For this review, take the finished solid that the model builds, in its own axes (mm). Face numbers are marked on the shaded views. A direction names the side the tool comes from. Give positions to 0.01 mm unless a question says otherwise; leave off trailing zeros. Order: outer loops, then holes, each group sorted by start corner. A loop starts at its lowest first (then second) coordinate and runs counter-clockwise, first axis right, second up. Notation, with made-up numbers: M 41.25,74.25 L 62.25,74.25 A6 ccw 62.25,79.25 Z; hole C 25,53 d3. An arc over 180 degrees is marked long. Answer as CSV lines item,"result". Start each with the question number.
1. For line 1 along Z through (x, y) = (18, -24); line 2 along Y through (x, z) = (18, 5); line 3 along Z through (x, y) = (-8.5, 7), list the stretches that pass through material, from the lowest coordinate up.
2. We need section D-D, the plane y = 27.5. Give the boundary of the cut face in (x, z).
3. Machinability: for the marked faces 5, 6 and 7, which of the approach directions +Z, -Z, +X, -X, +Y, -Y give a long, thin tool a straight path to every point of the face, cutting with its end or side? Answer none if there is none.
4. We need section C-C, the plane z = 5. Give the boundary of the cut face in (x, y), and give its area (3 significant figures).
5. Mouldability with a two-part tool opening along Z and no side actions: class the marked faces 1, 2, 3 and 4 as pulls with the +Z half, pulls with the -Z half, needs draft (parallel to the pull), parting line crosses it, or undercut.
6. We need section A-A, the plane x = 18. Give the boundary of the cut face in (y, z).
7. We need section B-B, the plane x = -14.5. Give the boundary of the cut face in (y, z), and give its area (3 significant figures).
8. Clearance check with flat-ended pins moving along their axes: P1, Ø3.5, axis at x = 9.5, z = 12, coming from the +Y side; P2, Ø2, axis at y = -2.5, z = -18.5, coming from the -X side; P3, Ø5, axis at x = 22.5, z = -16.5, coming from the +Y side; P4, Ø10, axis at x = -2.5, y = -10, coming from the +Z side. State where each tip first meets the part, or that it passes through.
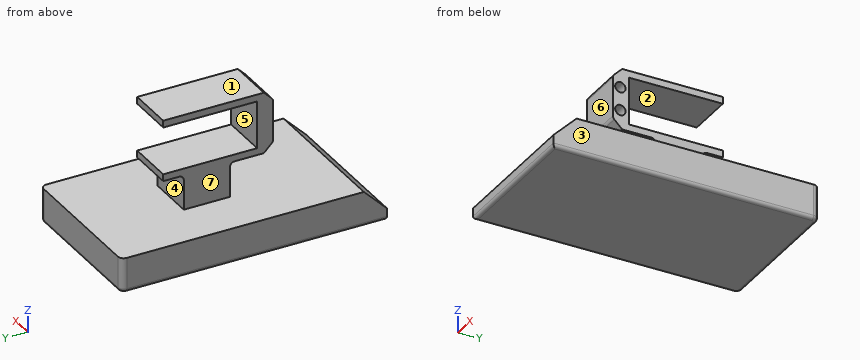
from build123d import *

# Parameters (mm, degrees)
SKETCH1_R            = 2.25
BOSS_EXTRUDE1_DEPTH  = 20
SKETCH2_R            = 2.25
BOSS_EXTRUDE2_DEPTH  = 10
SKETCH4_W            = 26.5
SKETCH4_H            = 2.5
CUT_EXTRUDE1_DEPTH   = 39.17921555
CHAMFER2_SIZE        = 4
CHAMFER3_SIZE        = 4
FILLET4_R            = 2
SKETCH7_W            = 15
SKETCH7_H            = 20
BOSS_EXTRUDE5_DEPTH  = 20
FILLET6_R            = 2
SKETCH13_R           = 2.25
BOSS_EXTRUDE8_DEPTH  = 20
CUT_EXTRUDE2_DEPTH   = 45.021614009
BOSS_EXTRUDE9_START  = -10
SKETCH14_R           = 2.25
BOSS_EXTRUDE9_DEPTH  = 10
BOSS_EXTRUDE10_START = 0.4
SKETCH15_R           = 2.25
BOSS_EXTRUDE10_DEPTH = 0.4
SKETCH16_W           = 63
SKETCH16_H           = 115
BOSS_EXTRUDE11_DEPTH = 15
CHAMFER4_SIZE        = 10
FILLET7_R            = 2.5
FILLET8_R            = 1.5


with BuildPart() as part:
    # Sketch1 → Boss-Extrude1 (new body)
    with BuildSketch(Plane(origin=(0, 0, 0), x_dir=(0, 0, -1), z_dir=(1, 0, 0))):
        Polygon((10.25, -20.3), (13.25, -20.3), (13.25, 29.7), (-13.25, 29.7), (-13.25, -20.3), (-10.25, -20.3), (-10.25, 20.3), (10.25, 20.3), align=None)
        with Locations((5, 24)):
            Circle(SKETCH1_R, mode=Mode.SUBTRACT)
        with Locations((-5, 24)):
            Circle(SKETCH1_R, mode=Mode.SUBTRACT)
    extrude(amount=BOSS_EXTRUDE1_DEPTH)

    # Sketch2 → Boss-Extrude2 (add)
    with BuildSketch(Plane.ZY):
        with Locations((-5, 24)):
            Circle(SKETCH2_R)
        with Locations((5, 24)):
            Circle(SKETCH2_R)
    extrude(amount=-BOSS_EXTRUDE2_DEPTH)

    # Sketch4 → Cut-Extrude1 (cut, through all)
    with BuildSketch(Plane(origin=(20, 0, 0), x_dir=(0, 0, -1), z_dir=(1, 0, 0))):
        with Locations((0, 28.45)):
            Rectangle(SKETCH4_W, SKETCH4_H)
    extrude(amount=-CUT_EXTRUDE1_DEPTH, mode=Mode.SUBTRACT)

    # Chamfer2
    chamfer2_edges = [part.edges().sort_by_distance(p)[0] for p in [
        (10, 27.2, -13.25),
    ]]
    chamfer(chamfer2_edges, length=CHAMFER2_SIZE)

    # Chamfer3
    chamfer3_edges = [part.edges().sort_by_distance(p)[0] for p in [
        (10, 27.2, 13.25),
    ]]
    chamfer(chamfer3_edges, length=CHAMFER3_SIZE)

    # Fillet4
    fillet4_edges = [part.edges().sort_by_distance(p)[0] for p in [
        (10, 27.2, -9.25),
        (10, 27.2, 9.25),
    ]]
    fillet(fillet4_edges, radius=FILLET4_R)

    # Sketch7 → Boss-Extrude5 (add)
    with BuildSketch(Plane(origin=(20, 0, 0), x_dir=(0, 0, -1), z_dir=(1, 0, 0))):
        with Locations((20.75, 1.423218073)):
            Rectangle(SKETCH7_W, SKETCH7_H)
    extrude(amount=-BOSS_EXTRUDE5_DEPTH)

    # Fillet6
    fillet6_edges = [part.edges().sort_by_distance(p)[0] for p in [
        (10, -8.576781927, -13.25),
        (10, 11.423218073, -13.25),
    ]]
    fillet(fillet6_edges, radius=FILLET6_R)

    # Sketch13 → Boss-Extrude8 (add)
    with BuildSketch(Plane(origin=(20, 0, 0), x_dir=(0, 0, -1), z_dir=(1, 0, 0))):
        with BuildLine():
            Line((-13.25, -23.2), (-9.835786438, -26.614213562))
            ThreePointArc((-9.835786438, -26.614213562), (-9.18693974, -27.047759065), (-8.421572875, -27.2))
            Line((-8.421572875, -27.2), (8.421572875, -27.2))
            ThreePointArc((8.421572875, -27.2), (9.18693974, -27.047759065), (9.835786438, -26.614213562))
            Line((9.835786438, -26.614213562), (13.25, -23.2))
            Line((13.25, -23.2), (13.25, -20.3))
            Line((13.25, -20.3), (-13.25, -20.3))
            Line((-13.25, -20.3), (-13.25, -23.2))
        make_face()
        with Locations((5, -24)):
            Circle(SKETCH13_R, mode=Mode.SUBTRACT)
        with Locations((-5, -24)):
            Circle(SKETCH13_R, mode=Mode.SUBTRACT)
    extrude(amount=-BOSS_EXTRUDE8_DEPTH)

    # Sketch12 → Cut-Extrude2 (cut, through all)
    with BuildSketch(Plane(origin=(20, 0, 0), x_dir=(0, 0, -1), z_dir=(1, 0, 0))):
        with BuildLine():
            Line((13.25, 23.2), (9.835786438, 26.614213562))
            ThreePointArc((9.835786438, 26.614213562), (9.18693974, 27.047759065), (8.421572875, 27.2))
            Line((8.421572875, 27.2), (-8.421572875, 27.2))
            ThreePointArc((-8.421572875, 27.2), (-9.18693974, 27.047759065), (-9.835786438, 26.614213562))
            Line((-9.835786438, 26.614213562), (-13.25, 23.2))
            Line((-13.25, 23.2), (-13.25, 20.3))
            Line((-13.25, 20.3), (13.25, 20.3))
            Line((13.25, 20.3), (13.25, 23.2))
        make_face()
    extrude(amount=-CUT_EXTRUDE2_DEPTH, mode=Mode.SUBTRACT)

    # Sketch14 → Boss-Extrude9 (add)
    with BuildSketch(Plane.ZY.offset(BOSS_EXTRUDE9_START)):
        with Locations(Location((-5, -24, 0), (0, 0, 180))):
            Circle(SKETCH14_R)
        with Locations(Location((5, -24, 0), (0, 0, 180))):
            Circle(SKETCH14_R)
    extrude(amount=BOSS_EXTRUDE9_DEPTH)

    # Sketch15 → Boss-Extrude10 (add)
    with BuildSketch(Plane(origin=(20, 0, 0), x_dir=(0, 0, -1), z_dir=(1, 0, 0)).offset(BOSS_EXTRUDE10_START)):
        with BuildLine():
            Line((-10.25, 20.3), (-13.25, 20.3))
            Line((-13.25, 20.3), (-13.25, -23.2))
            Line((-13.25, -23.2), (-9.835786438, -26.614213562))
            ThreePointArc((-9.835786438, -26.614213562), (-9.18693974, -27.047759065), (-8.421572875, -27.2))
            Line((-8.421572875, -27.2), (8.421572875, -27.2))
            ThreePointArc((8.421572875, -27.2), (9.18693974, -27.047759065), (9.835786438, -26.614213562))
            Line((9.835786438, -26.614213562), (13.25, -23.2))
            Line((13.25, -23.2), (13.25, -10.576781927))
            ThreePointArc((13.25, -10.576781927), (13.835786438, -9.162568365), (15.25, -8.576781927))
            Line((15.25, -8.576781927), (28.25, -8.576781927))
            Line((28.25, -8.576781927), (28.25, 11.423218073))
            Line((28.25, 11.423218073), (15.25, 11.423218073))
            ThreePointArc((15.25, 11.423218073), (13.835786438, 12.00900451), (13.25, 13.423218073))
            Line((13.25, 13.423218073), (13.25, 20.3))
            Line((13.25, 20.3), (10.25, 20.3))
            Line((10.25, 20.3), (10.25, -20.3))
            Line((10.25, -20.3), (-10.25, -20.3))
            Line((-10.25, -20.3), (-10.25, 20.3))
        make_face()
        with Locations((5, -24)):
            Circle(SKETCH15_R, mode=Mode.SUBTRACT)
        with Locations((-5, -24)):
            Circle(SKETCH15_R, mode=Mode.SUBTRACT)
    extrude(amount=-BOSS_EXTRUDE10_DEPTH)

    # Sketch16 → Boss-Extrude11 (add)
    with BuildSketch(Plane(origin=(0, 0, -28.25), x_dir=(-1, 0, 0), z_dir=(0, 0, -1))):
        with Locations((-10.2, -7.2)):
            Rectangle(SKETCH16_W, SKETCH16_H)
    extrude(amount=BOSS_EXTRUDE11_DEPTH)

    # Chamfer4
    chamfer4_edges = [part.edges().sort_by_distance(p)[0] for p in [
        (10.2, -64.7, -28.25),
    ]]
    chamfer(chamfer4_edges, length=CHAMFER4_SIZE)

    # Fillet7
    fillet7_edges = [part.edges().sort_by_distance(p)[0] for p in [
        (41.7, 50.3, -35.75),
        (-21.3, 50.3, -35.75),
    ]]
    fillet(fillet7_edges, radius=FILLET7_R)

    # Fillet8
    fillet8_edges = [part.edges().sort_by_distance(p)[0] for p in [
        (10.2, -64.7, -43.25),
        (-21.3, -8.45, -43.25),
        (10.2, 50.3, -43.25),
        (41.7, -8.45, -43.25),
        (40.967766953, 49.567766953, -43.25),
        (-20.567766953, 49.567766953, -43.25),
    ]]
    fillet(fillet8_edges, radius=FILLET8_R)


solid = part.part
Result set:
1,line 1,"-43.25 to -28.25, -12.45 to -7.25, -2.75 to 2.75, 7.25 to 12.45"
1,line 2,"-27.2 to -26.25, -21.75 to -20.3"
1,line 3,"-43.25 to -28.25"
2,outline,"M -21.3,-41.75 A1.5 ccw -19.8,-43.25 L 40.2,-43.25 A1.5 ccw 41.7,-41.75 L 41.7,-28.25 L -21.3,-28.25 Z"
3,face 5,"+X, -X, +Y"
3,face 6,"+Z, +X, -X, -Y"
3,face 7,"+Z, -X, +Y, -Y"
4,outline,"M 0,-27.2 L 20.4,-27.2 L 20.4,-26.25 L 10,-26.25 L 10,-21.75 L 20.4,-21.75 L 20.4,-20.3 L 0,-20.3 Z"
4,area,"94.0 mm2"
5,face 1,"pulls with the +Z half"
5,face 2,"undercut"
5,face 3,"needs draft"
5,face 4,"undercut"
6,outline,"M -64.7,-41.75 A1.5 ccw -63.2,-43.25 L 48.8,-43.25 A1.5 ccw 50.3,-41.75 L 50.3,-28.25 L 11.42,-28.25 L 11.42,-15.25 A2 cw 13.42,-13.25 L 20.3,-13.25 L 20.3,-10.25 L -20.3,-10.25 L -20.3,10.25 L 20.3,10.25 L 20.3,13.25 L -23.2,13.25 L -26.61,9.84 A2 ccw -27.2,8.42 L -27.2,-8.42 A2 ccw -26.61,-9.84 L -23.2,-13.25 L -10.58,-13.25 A2 cw -8.58,-15.25 L -8.58,-28.25 L -54.7,-28.25 L -64.7,-38.25 Z; hole C -24,-5 d4.5; hole C -24,5 d4.5"
7,outline,"M -64.7,-41.75 A1.5 ccw -63.2,-43.25 L 48.8,-43.25 A1.5 ccw 50.3,-41.75 L 50.3,-28.25 L -54.7,-28.25 L -64.7,-38.25 Z"
7,area,"1,670 mm2"
8,P1,"y = 20.3"
8,P2,"x = 0"
8,P3,"y = 11.43"
8,P4,"z = 13.25"
